Check sheet for the drawn part. Datum: minimum x, y, z corner. Units: mm. A direction names the side the tool comes from. Coordinates: 2 decimals unless noted, no trailing zeros. Write each loop counter-clockwise with the first axis right and the second up, starting at its lowest first coordinate (ties: lowest second). Pieces come first, ordered by that corner, then holes. Notation, with made-up numbers: (-19.5, 61) -> (38.5, 61) arc R12 cw to (38.5, 73) -> close; hole circle Ø1 at (50, 82.25). An arc over 180 degrees is marked (long way). Answer in a Markdown table with one row per item. Add a question column.
1. Cross-section at C-C on z = 8. Record the cut outline in (x, y).
2. Depth check by flat-ended pin: P1, Ø6, axis at x = 37, z = 20.5, coming from the -Y side; P2, Ø3.5, axis at x = 33, y = 62.3, coming from the -Z side. Enter the tip coordinate at first touch or a pass-through.
3. Cross-section at A-A on y = 66. Record the cut outline in (x, z).
4. Scan lines: L1, parallel to Y at x = 9, z = 0.8 (3 decimals); L2, parallel to X at y = 38.3, z = 0.9 (3 decimals); L3, parallel to Z at x = 7.5, y = 52. Record each from-to range of solid material in increasing order. Write a range as from..to.
5. Mould release check, pull along X, two halves, no side actions. Record for the marked faces 1, 2, 3 and 4: pulls with the +X half, pulls with the -X half, needs draft (parallel to the pull), parting line crosses it, or undercut.
6. Set-up check for the marked faces 5 and 6: record each of +Z, -Z, +X, -X, +Y, -Y from which the full face is reachable in a straight line by a thin tool's end or side.
7. Cross-section at D-D on y = 26.3. Record the cut outline in (x, z) (3 decimals).
8. Cross-section at B-B on x = 21. Record the cut outline in (y, z) (3 decimals), and give its area (3 significant figures).
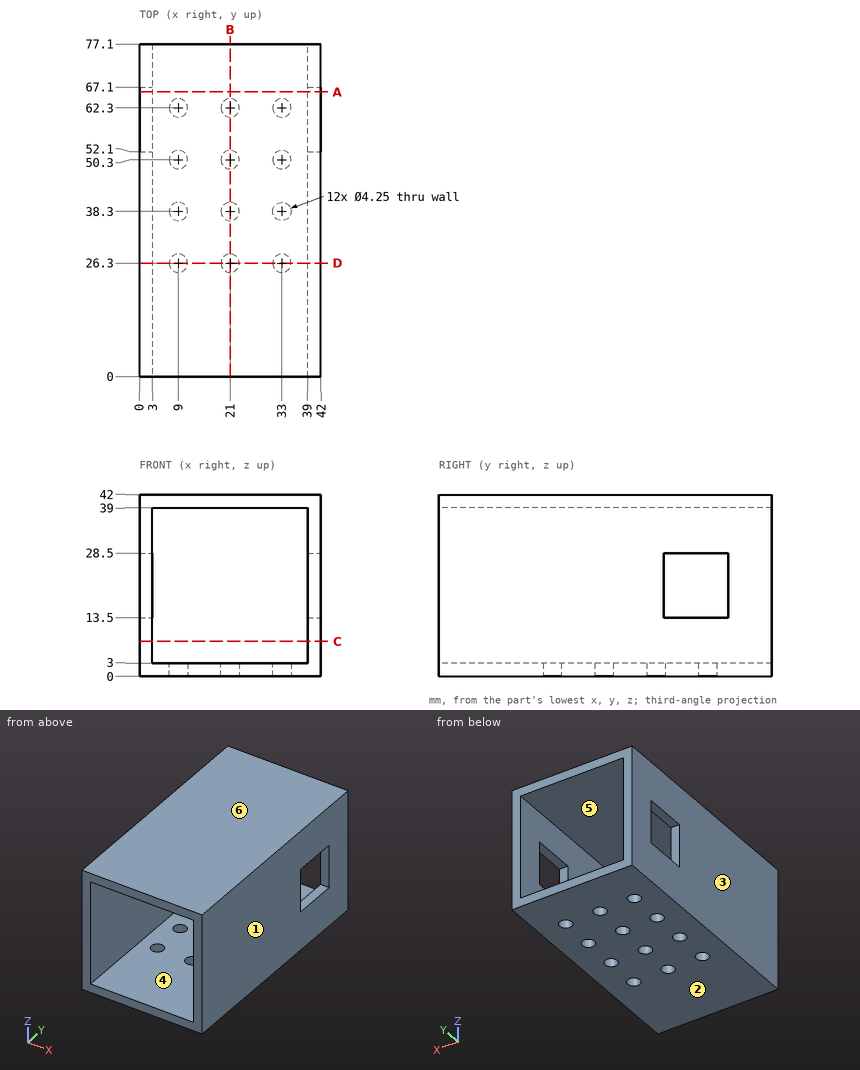
Results found:
| question | item | result |
|---|---|---|
| 1 | outline | (0, 0) -> (3, 0) -> (3, 77.1) -> (0, 77.1) -> close; (39, 0) -> (42, 0) -> (42, 77.1) -> (39, 77.1) -> close |
| 2 | P1 | stops at y = 0 |
| 2 | P2 | stops at z = 39 |
| 3 | outline | (0, 0) -> (42, 0) -> (42, 13.5) -> (39, 13.5) -> (39, 3) -> (3, 3) -> (3, 13.5) -> (0, 13.5) -> close; (0, 28.5) -> (3, 28.5) -> (3, 39) -> (39, 39) -> (39, 28.5) -> (42, 28.5) -> (42, 42) -> (0, 42) -> close |
| 4 | L1 | y = 0..24.175, 28.425..36.175, 40.425..48.175, 52.425..60.175, 64.425..77.1 |
| 4 | L2 | x = 0..6.875, 11.125..18.875, 23.125..30.875, 35.125..42 |
| 4 | L3 | z = 0..3, 39..42 |
| 5 | face 1 | pulls with the +X half |
| 5 | face 2 | needs draft |
| 5 | face 3 | pulls with the -X half |
| 5 | face 4 | undercut |
| 6 | face 5 | +Y, -Y |
| 6 | face 6 | +Z, +X, -X, +Y, -Y |
| 7 | outline | (0, 0) -> (6.875, 0) -> (6.875, 3) -> (3, 3) -> (3, 39) -> (39, 39) -> (39, 3) -> (35.125, 3) -> (35.125, 0) -> (42, 0) -> (42, 42) -> (0, 42) -> close; (11.125, 0) -> (18.875, 0) -> (18.875, 3) -> (11.125, 3) -> close; (23.125, 0) -> (30.875, 0) -> (30.875, 3) -> (23.125, 3) -> close |
| 8 | outline | (0, 0) -> (24.175, 0) -> (24.175, 3) -> (0, 3) -> close; (0, 39) -> (77.1, 39) -> (77.1, 42) -> (0, 42) -> close; (28.425, 0) -> (36.175, 0) -> (36.175, 3) -> (28.425, 3) -> close; (40.425, 0) -> (48.175, 0) -> (48.175, 3) -> (40.425, 3) -> close; (52.425, 0) -> (60.175, 0) -> (60.175, 3) -> (52.425, 3) -> close; (64.425, 0) -> (77.1, 0) -> (77.1, 3) -> (64.425, 3) -> close |
| 8 | area | 412 mm^2 |
